Can you work these out from the model? Positions are in its coordinate system, mm. Face numbers are marked on the shaded views. A direction names the side the tool comes from. Round coordinates to 2 decimals unless told otherwise and drop trailing zeros. Write each loop counter-clockwise with the first axis right and the second up, starting at its lowest first coordinate (ties: lowest second). Pieces come first, ordered by that corner, then holes. Notation, with made-up numbers: (79, 62) -> (115, 62) arc R10 cw to (115, 66) -> close; hole circle Ø10 at (63, 36.5). An arc over 180 degrees is marked (long way). Write item = value, one per line. Start each with the question number.
1) Imagine slicing it at B-B, the plane x = 2.5. Please give me the cut outline in (y, z).
2) Imagine slicing it at D-D, the plane y = 4. Please give me the cut outline in (x, z), then the cut area to 3 significant figures.
3) Thinking about a two-plate mould opening in Y: for the marked faces 3, 4 and 5, which applies, +Y half, -Y half, draft (parallel to the pull), parting line (faces both ways), or undercut?
4) Imagine slicing it at C-C, the plane y = 10. Please give me the cut outline in (x, z), then the cut area to 4 significant figures.
5) Imagine slicing it at A-A, the plane z = 5. Please give me the cut outline in (x, y), then the cut area to 3 significant figures.
6) I'm going to push flat-ended pins straight in: pin 1 (0.8 mm diameter, centred on x = 2, z = 5.5, fed in from +Y); pin 2 (0.8 mm diameter, centred on x = 2.5, z = 5, fed in from -Y); pin 3 (1.5 mm diameter, centred on x = 4.5, z = 4, fed in from -Y). Where does each tip first touch, or does it pass through?
7) For the marked faces 1 and 2, which set-ups out of +Z, -Z, +X, -X, +Y, -Y let a thin tool reach every point of the face, with its end or its side?
8) If I drill on line 1 (X direction, y = 10, z = 3.1); line 2 (Y direction, x = 2.5, z = 3.15); line 3 (Y direction, x = 4.1, z = 5), over which ranges is the centre line in solid material (lowest first)?
Autodesk Inventor part; units mm, degrees
ref_plane "YZ Plane" through (0, 0, 0) normal (1, 0, 0) x (0, 1, 0)
ref_plane "XZ Plane" through (0, 0, 0) normal (0, 1, 0) x (-1, 0, 0)
ref_plane "XY Plane" through (0, 0, 0) normal (0, 0, 1) x (1, 0, 0)
sketch "Skizze1" plane through (0, 0, 0) normal (0, 0, 1) x (1, 0, 0)
  line L0 (2, 0) -> (3, 0)
  line L1 (5, 2) -> (5, 48)
  line L2 (3, 50) -> (2, 50)
  line L3 (0, 48) -> (0, 2)
  arc A0 (5, 48) -> (3, 50) centre (3, 48) ccw
  arc A1 (3, 0) -> (5, 2) centre (3, 2) ccw
  arc A2 (0, 2) -> (2, 0) centre (2, 2) ccw
  arc A3 (2, 50) -> (0, 48) centre (2, 48) ccw
  point P0 (0, 0)
  point P1 (5, 50)
  point P2 (5, 0)
  point P3 (0, 50)
  dimension "d0" = 5
  dimension "d1" = 50
  dimension "d2" = 2
extrude "Extrusion1" add sketch "Skizze1" along normal blind 4
sketch "Skizze2" plane through (0, 0, 4) normal (0, 0, 1) x (1, 0, 0)
  line L0 (5, 2) -> (5, 48)
  line L1 (3, 50) -> (2, 50)
  line L2 (2, 0) -> (3, 0)
  line L3 (0, 48) -> (0, 2)
  line L4 (1, 42.5) -> (4, 42.5)
  line L5 (5, 41.5) -> (5, 38.5)
  line L6 (4, 37.5) -> (1, 37.5)
  line L7 (0, 38.5) -> (0, 41.5)
  line L8 (1, 12.5) -> (4, 12.5)
  line L9 (5, 11.5) -> (5, 8.5)
  line L10 (4, 7.5) -> (1, 7.5)
  line L11 (0, 8.5) -> (0, 11.5)
  arc A0 (5, 41.5) -> (4, 42.5) centre (4, 41.5) ccw
  arc A1 (4, 37.5) -> (5, 38.5) centre (4, 38.5) ccw
  arc A2 (0, 38.5) -> (1, 37.5) centre (1, 38.5) ccw
  arc A3 (1, 42.5) -> (0, 41.5) centre (1, 41.5) ccw
  arc A4 (5, 11.5) -> (4, 12.5) centre (4, 11.5) ccw
  arc A5 (4, 7.5) -> (5, 8.5) centre (4, 8.5) ccw
  arc A6 (0, 8.5) -> (1, 7.5) centre (1, 8.5) ccw
  arc A7 (1, 12.5) -> (0, 11.5) centre (1, 11.5) ccw
  point P0 (0, 0)
  point P1 (0, 42.5)
  point P2 (5, 37.5)
  point P3 (0, 12.5)
  point P4 (5, 7.5)
  dimension "d12" = 1
  dimension "d13" = 7.5
  dimension "d14" = 5
  dimension "d15" = 5
  dimension "d16" = 7.5
extrude "Extrusion2" add sketch "Skizze2" along normal blind 2.5 contours A5 L10 A6 L3 A7 L8 A4 L0 | A1 L6 A2 L3 A3 L4 A0 L0
hole "Bohrung2" at (2.5, 40, 0) direction (0, 0, 1) diameter 3 end through all countersink diameter 4 countersink angle 90
hole "Bohrung3" at (2.5, 10, 0) direction (0, 0, 1) diameter 3 end through all countersink diameter 4 countersink angle 90
equation "\"d15\" = d14"
equation "\"d16\" = d13"
equation "\"d26\" = 0.5 * d0"
equation "\"d27\" = 0.5 * d14"
equation "\"d36\" = 0.5 * d15"
properties part number "Halter"
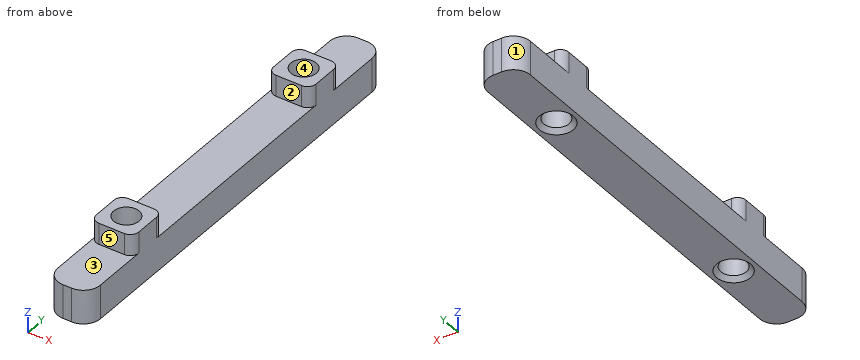
Reported:
q1.outline = (0, 0) -> (8, 0) -> (8.5, 0.5) -> (8.5, 6.5) -> (7.5, 6.5) -> (7.5, 4) -> (0, 4) -> close; (11.5, 0.5) -> (12, 0) -> (38, 0) -> (38.5, 0.5) -> (38.5, 6.5) -> (37.5, 6.5) -> (37.5, 4) -> (12.5, 4) -> (12.5, 6.5) -> (11.5, 6.5) -> close; (41.5, 0.5) -> (42, 0) -> (50, 0) -> (50, 4) -> (42.5, 4) -> (42.5, 6.5) -> (41.5, 6.5) -> close
q2.outline = (0, 0) -> (5, 0) -> (5, 4) -> (0, 4) -> close
q2.area = 20.0 mm²
q3.face_3 = draft
q3.face_4 = undercut
q3.face_5 = -Y half
q4.outline = (0, 0) -> (0.5, 0) -> (1, 0.5) -> (1, 6.5) -> (0, 6.5) -> close; (4, 0.5) -> (4.5, 0) -> (5, 0) -> (5, 6.5) -> (4, 6.5) -> close
q4.area = 12.75 mm²
q5.outline = (0, 8.5) arc R1 ccw to (1, 7.5) -> (4, 7.5) arc R1 ccw to (5, 8.5) -> (5, 11.5) arc R1 ccw to (4, 12.5) -> (1, 12.5) arc R1 ccw to (0, 11.5) -> close; (0, 38.5) arc R1 ccw to (1, 37.5) -> (4, 37.5) arc R1 ccw to (5, 38.5) -> (5, 41.5) arc R1 ccw to (4, 42.5) -> (1, 42.5) arc R1 ccw to (0, 41.5) -> close; hole circle Ø3 at (2.5, 10); hole circle Ø3 at (2.5, 40)
q5.area = 34.1 mm²
q6.pin_1 = 42.5
q6.pin_2 = 7.5
q6.pin_3 = 0.15
q7.face_1 = +Z, -Z, -X, +Y
q7.face_2 = +Z, +X, -X
q8.line_1 = 0 to 1, 4 to 5
q8.line_2 = 0 to 8.5, 11.5 to 38.5, 41.5 to 50
q8.line_3 = 7.51 to 12.49, 37.51 to 42.49
